For this review, take the finished solid that the model builds, in its own axes (mm). Face numbers are marked on the shaded views. Round coordinates to 2 decimals unless told otherwise and drop trailing zeros. Loops run counter-clockwise (first coordinate to the right, second up) from the corner with the lowest first, then second, coordinate; pieces in that order, holes last.
```python
from build123d import *

# Parameters (mm, degrees)
BOSS_EXTRUDE1_DEPTH = 15
SKETCH2_W           = 138
SKETCH2_H           = 93.2
CUT_EXTRUDE1_DEPTH  = 11
SKETCH3_W           = 2.5
SKETCH3_H           = 82.2
SKETCH3_W_2         = 127
SKETCH3_H_2         = 2.5
CUT_EXTRUDE2_DEPTH  = 11
SKETCH7_W           = 123
SKETCH7_H           = 7
CUT_EXTRUDE6_DEPTH  = 2
SKETCH8_W           = 123
SKETCH8_H           = 5
CUT_EXTRUDE7_DEPTH  = 10


with BuildPart() as part:
    # Sketch1 → Boss-Extrude1 (new body)
    with BuildSketch(Plane(origin=(0, 0, 0), x_dir=(1, 0, 0), z_dir=(0, 1, 0))):
        with BuildLine():
            Line((-69.5, -49.1), (69.5, -49.1))
            ThreePointArc((69.5, -49.1), (70.914213562, -48.514213562), (71.5, -47.1))
            Line((71.5, -47.1), (71.5, 47.1))
            ThreePointArc((71.5, 47.1), (70.914213562, 48.514213562), (69.5, 49.1))
            Line((69.5, 49.1), (-69.5, 49.1))
            ThreePointArc((-69.5, 49.1), (-70.914213562, 48.514213562), (-71.5, 47.1))
            Line((-71.5, 47.1), (-71.5, -47.1))
            ThreePointArc((-71.5, -47.1), (-70.914213562, -48.514213562), (-69.5, -49.1))
        make_face()
    extrude(amount=BOSS_EXTRUDE1_DEPTH)

    # Sketch2 → Cut-Extrude1 (cut)
    with BuildSketch(Plane(origin=(0, 15, 0), x_dir=(1, 0, 0), z_dir=(0, 1, 0))):
        Rectangle(SKETCH2_W, SKETCH2_H)
    extrude(amount=-CUT_EXTRUDE1_DEPTH, mode=Mode.SUBTRACT)

    # Sketch3 → Cut-Extrude2 (cut)
    with BuildSketch(Plane(origin=(0, 15, 0), x_dir=(1, 0, 0), z_dir=(0, 1, 0))):
        with Locations((-70.25, 0)):
            Rectangle(SKETCH3_W, SKETCH3_H)
        with Locations((0, 47.85)):
            Rectangle(SKETCH3_W_2, SKETCH3_H_2)
        with Locations((70.25, 0)):
            Rectangle(SKETCH3_W, SKETCH3_H)
        with Locations((0, -47.85)):
            Rectangle(SKETCH3_W_2, SKETCH3_H_2)
    extrude(amount=-CUT_EXTRUDE2_DEPTH, mode=Mode.SUBTRACT)

    # Sketch7 → Cut-Extrude6 (cut)
    with BuildSketch(Plane(origin=(0, 4, 0), x_dir=(1, 0, 0), z_dir=(0, 1, 0))):
        with Locations((0, 0.9)):
            Rectangle(SKETCH7_W, SKETCH7_H)
        with Locations((0, 24.1)):
            Rectangle(SKETCH7_W, SKETCH7_H)
        with Locations((0, -24.1)):
            Rectangle(SKETCH7_W, SKETCH7_H)
    extrude(amount=-CUT_EXTRUDE6_DEPTH, mode=Mode.SUBTRACT)

    # Sketch8 → Cut-Extrude7 (cut)
    with BuildSketch(Plane(origin=(0, 2, 0), x_dir=(1, 0, 0), z_dir=(0, 1, 0))):
        with Locations((0, 0.9)):
            Rectangle(SKETCH8_W, SKETCH8_H)
        with Locations((0, 24.1)):
            Rectangle(SKETCH8_W, SKETCH8_H)
        with Locations((0, -24.1)):
            Rectangle(SKETCH8_W, SKETCH8_H)
    extrude(amount=-CUT_EXTRUDE7_DEPTH, mode=Mode.SUBTRACT)


solid = part.part
```
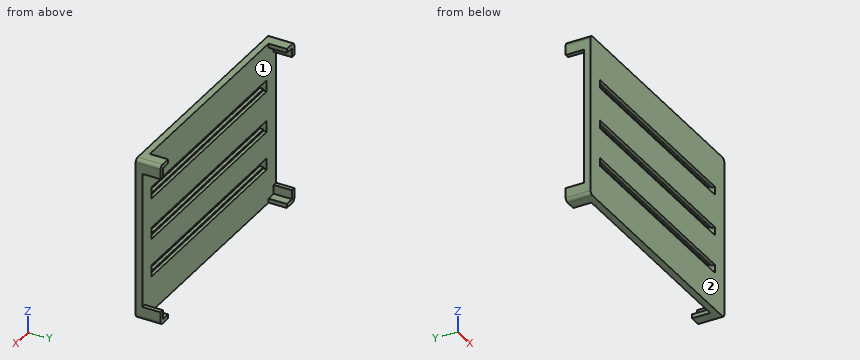
(1) Add section B-B (y = 9.25). Give the boundary of the cut face in (x, z).
(2) The part is to be moulded in two halves that separate along X. For the marked faces 1 and 2, say which applies: pulls with the +X half, pulls with the -X half, needs draft (parallel to the pull), parting line crosses it, or undercut.
(3) Add section A-A (x = -57). Give the boundary of the cut face in (y, z).
(4) Insertion check: pin 1 Ø2 at (x, z) = (54.5, 9.5) entering from -Y; pin 2 Ø1.2 at (x, y) = (70.5, 9.5) entering from -Z; pin 3 Ø0.8 at (x, y) = (-70.5, 7) entering from +Z; pin 4 Ø0.5 at (x, z) = (-22.5, -21.5) entering from +Y. Each pin has a flat end and moves straight along its axis. Give the tip position at first contact, or say it passes through.
(5) For L1, parallel to Z at x = 46, y = 3.25; L2, parallel to X at y = 1, z = -2; L3, parallel to Y at x = 26.5, z = 2, list the stretches that pass through material, from the lowest coordinate up.
(6) Add section C-C (z = -38.5). Give the boundary of the cut face in (x, y).
Outcome:
1. outline: (-71.5, -47.1) arc R2 ccw to (-69.5, -49.1) - (-63.5, -49.1) - (-63.5, -46.6) - (-69, -46.6) - (-69, -41.1) - (-71.5, -41.1) - close; (-71.5, 41.1) - (-69, 41.1) - (-69, 46.6) - (-63.5, 46.6) - (-63.5, 49.1) - (-69.5, 49.1) arc R2 ccw to (-71.5, 47.1) - close; (63.5, -49.1) - (69.5, -49.1) arc R2 ccw to (71.5, -47.1) - (71.5, -41.1) - (69, -41.1) - (69, -46.6) - (63.5, -46.6) - close; (63.5, 46.6) - (69, 46.6) - (69, 41.1) - (71.5, 41.1) - (71.5, 47.1) arc R2 ccw to (69.5, 49.1) - (63.5, 49.1) - close
2. face 1: undercut
2. face 2: needs draft
3. outline: (0, -49.1) - (4, -49.1) - (4, -27.6) - (2, -27.6) - (2, -26.6) - (0, -26.6) - close; (0, -21.6) - (2, -21.6) - (2, -20.6) - (4, -20.6) - (4, -4.4) - (2, -4.4) - (2, -3.4) - (0, -3.4) - close; (0, 1.6) - (2, 1.6) - (2, 2.6) - (4, 2.6) - (4, 20.6) - (2, 20.6) - (2, 21.6) - (0, 21.6) - close; (0, 26.6) - (2, 26.6) - (2, 27.6) - (4, 27.6) - (4, 49.1) - (0, 49.1) - close
4. pin 1: stops at y = 0
4. pin 2: stops at z = -49.06
4. pin 3: stops at z = 49.01
4. pin 4: stops at y = 2
5. L1: z = -49.1 to -27.6, -20.6 to -4.4, 2.6 to 20.6, 27.6 to 49.1
5. L2: x = -71.5 to -61.5, 61.5 to 71.5
5. L3: y = 0 to 2
6. outline: (-71.5, 0) - (71.5, 0) - (71.5, 4) - (-71.5, 4) - close
